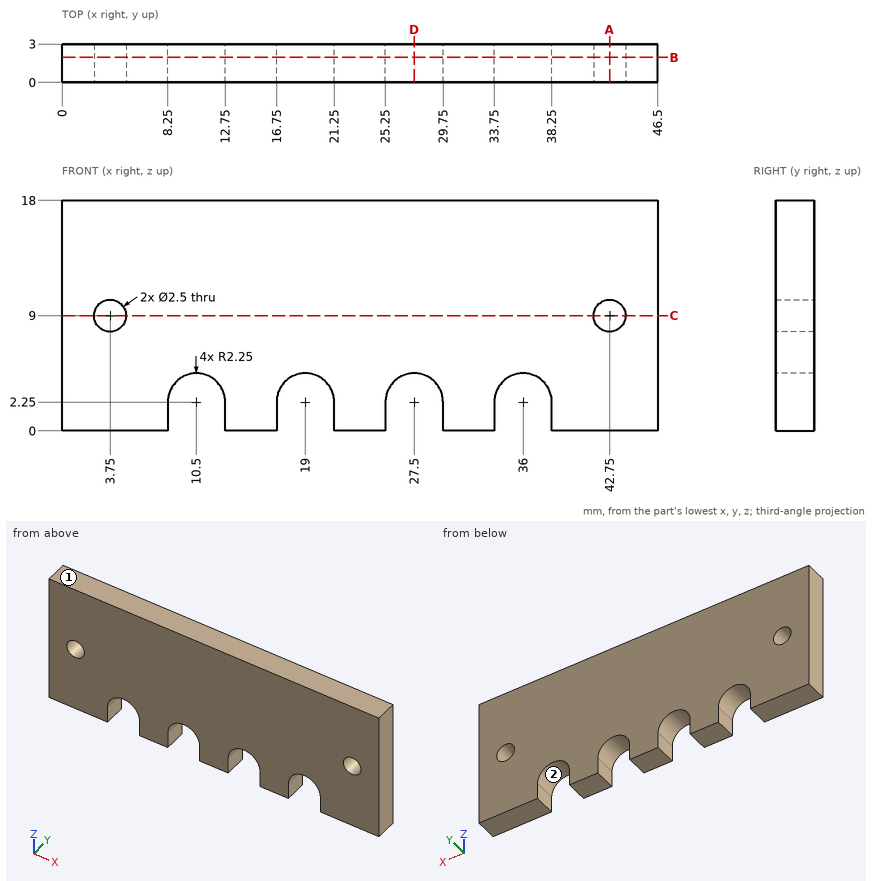
Study the drawing (mm; zero at the part's minimum x, y, z) and answer. Coordinates: 2 decimals unless noted, no trailing zeros. Write each loop counter-clockwise with the first axis right and the second up, starting at its lowest first coordinate (ties: lowest second). Pieces come first, ordered by that corner, then holes. Notation, with made-up numbers: (50, 38.25) - (74, 38.25) arc R25 ccw to (74, 52.25) - close; hole circle Ø6 at (76.5, 56.5). An arc over 180 degrees is marked (long way). One line per item, written item: value.
1) Find section A-A (x = 42.75). Give the vertices of the cut face in (y, z).
Geometry check:
outline: (0, 0) - (3, 0) - (3, 7.75) - (0, 7.75) - close; (0, 10.25) - (3, 10.25) - (3, 18) - (0, 18) - close
2) This flat-tipped pin is pushed along its axis until it touches: pin 1 Ø10 at (x, z) = (31, 11.5) entering from -Y. Where does it stop, or does it pass through?
Geometry check:
pin 1: stops at y = 0
3) Find section B-B (y = 1.95). Give the vertices of the cut face in (x, z), and give its area (3 significant figures).
Geometry check:
outline: (0, 0) - (8.25, 0) - (8.25, 2.25) arc R2.25 cw to (12.75, 2.25) - (12.75, 0) - (16.75, 0) - (16.75, 2.25) arc R2.25 cw to (21.25, 2.25) - (21.25, 0) - (25.25, 0) - (25.25, 2.25) arc R2.25 cw to (29.75, 2.25) - (29.75, 0) - (33.75, 0) - (33.75, 2.25) arc R2.25 cw to (38.25, 2.25) - (38.25, 0) - (46.5, 0) - (46.5, 18) - (0, 18) - close; hole circle Ø2.5 at (3.75, 9); hole circle Ø2.5 at (42.75, 9)
area: 755 mm2
4) Consider line 1 along X through (y, z) = (1.7, 9); line 2 along X through (y, z) = (2.6, 9.5); line 3 along X through (y, z) = (2.3, 3). Determine where each line is inside the solid, lowest interval first. Write a range as from..to.
Geometry check:
line 1: x = 0..2.5, 5..41.5, 44..46.5
line 2: x = 0..2.6, 4.9..41.6, 43.9..46.5
line 3: x = 0..8.38, 12.62..16.88, 21.12..25.38, 29.62..33.88, 38.12..46.5
5) Find section D-D (x = 27.5). Give the vertices of the cut face in (y, z), and give its area (3 significant figures).
Geometry check:
outline: (0, 4.5) - (3, 4.5) - (3, 18) - (0, 18) - close
area: 40.5 mm2
6) For a pull along X with two mould halves and no side action, classify the marked faces 1 and 2 as pulls with the +X half, pulls with the -X half, needs draft (parallel to the pull), parting line crosses it, or undercut.
Geometry check:
face 1: needs draft
face 2: undercut
7) Find section C-C (z = 9). Give the vertices of the cut face in (x, y), and give its area (4 significant figures).
Geometry check:
outline: (0, 0) - (2.5, 0) - (2.5, 3) - (0, 3) - close; (5, 0) - (41.5, 0) - (41.5, 3) - (5, 3) - close; (44, 0) - (46.5, 0) - (46.5, 3) - (44, 3) - close
area: 124.5 mm2
